```python
from build123d import *

# Parameters (mm, degrees)
F0_W      = 50.8
F0_H      = 50.8
F1_DEPTH  = 63.5
F3_DEPTH  = 12.7
F5_DEPTH  = 6.35
F6_DEPTH  = 50.8
F8_DEPTH  = 50.8
F10_DEPTH = 12.7


with BuildPart() as f1:
    # F0 (on Top) → F1 (new body)
    with BuildSketch(Plane.XY):
        Rectangle(F0_W, F0_H)
    extrude(amount=F1_DEPTH)

    # F2 (on face) → F3 (join)
    with BuildSketch(Plane.YZ.offset(25.4)):
        Polygon((-14.0506572952, 63.5), (0, 76.2), (0, 86.4714240594), (-36.0647195239, 53.8735228844), (-30.9551258806, 48.2205190104), (-25.4, 53.2416434461), (-25.4, 63.5), align=None)
        Polygon((-25.4, 53.2416434461), (-14.0506572952, 63.5), (-25.4, 63.5), align=None)
        Polygon((0, 86.4714240594), (0, 76.2), (14.0506572952, 63.5), (25.4, 63.5), (25.4, 53.2416434461), (31.0640838699, 48.1220349014), (36.1736775133, 53.7750387754), align=None)
        Polygon((25.4, 63.5), (14.0506572952, 63.5), (25.4, 53.2416434461), align=None)
    extrude(amount=F3_DEPTH)

    # F4 (on face) → F5 (join)
    with BuildSketch(Plane.YZ.offset(25.4)):
        Polygon((-14.0506572952, 63.5), (-25.4, 53.2416434461), (0, 25.1403288557), (25.4, 53.2416434461), (14.0506572952, 63.5), align=None)
        Polygon((0, 76.2), (-14.0506572952, 63.5), (14.0506572952, 63.5), align=None)
    extrude(amount=F5_DEPTH)

    # F6 (add): faces of the model
    f6_faces = [f1.faces().sort_by_distance(p)[0] for p in [
        (25.4, 0.0499832571, 67.5742219927),
        (25.4, 0.0499832571, 67.5742219927),
        (25.4, 0.0499832571, 67.5742219927),
    ]]
    extrude(f6_faces, amount=F6_DEPTH)

    # F7 (on face) → F8 (cut)
    with BuildSketch(Plane.YZ.offset(31.75)):
        with BuildLine():
            Line((-6.35, 53.2416434461), (6.35, 53.2416434461))
            ThreePointArc((6.35, 53.2416434461), (0, 59.5916434461), (-6.35, 53.2416434461))
        make_face()
        with BuildLine():
            ThreePointArc((-6.35, 53.2416434461), (0, 46.8916434461), (6.35, 53.2416434461))
            Line((6.35, 53.2416434461), (-6.35, 53.2416434461))
        make_face()
    extrude(amount=-F8_DEPTH, mode=Mode.SUBTRACT)

    # F9 (on face) → F10 (join)
    with BuildSketch(Plane.YZ.offset(31.75)):
        with BuildLine():
            ThreePointArc((1.27, 41.6503288557), (-0.8980256121, 42.5483544678), (0, 40.3803288557))
            ThreePointArc((0, 40.3803288557), (0.8980256121, 40.7523032436), (1.27, 41.6503288557))
        make_face()
    extrude(amount=F10_DEPTH)


solid = f1.part
```
Build history of the part. All positions in model axes, mm. A direction names the side the tool comes from. Coordinates: 2 decimals unless noted, no trailing zeros. Write each loop counter-clockwise with the first axis right and the second up, starting at its lowest first coordinate (ties: lowest second). Pieces come first, ordered by that corner, then holes.
1. Band-saw the part on D-D, the plane y = 9.5. Give the cut face in (x, z), and give its area (3 significant figures).
Answer block:
outline: (-25.4, 0) - (25.4, 0) - (25.4, 35.65) - (31.75, 35.65) - (31.75, 67.61) - (38.1, 67.61) - (38.1, 77.88) - (-25.4, 77.88) - close
area: 4,290 mm2
2. Drop flat-ended pins along their axis: pin 1 (1 mm diameter, centred on y = 5, z = 67, fed in from +X); pin 2 (10 mm diameter, centred on x = 4, z = 35, fed in from +Y); pin 3 (15 mm diameter, centred on y = -7, z = 63, fed in from +X). Give the stop position or say it passes through.
Answer block:
pin 1: stops at x = 31.75
pin 2: stops at y = 25.4
pin 3: stops at x = 38.1
3. Band-saw the part on A-A, the plane x = -15. Give the cut face in (y, z).
Answer block:
outline: (-36.06, 53.87) - (-30.96, 48.22) - (-25.4, 53.24) - (-25.4, 0) - (25.4, 0) - (25.4, 53.24) - (31.06, 48.12) - (36.17, 53.78) - (0, 86.47) - close; hole circle Ø12.7 at (0, 53.24)
4. Band-saw the part on B-B, the plane z = 31. Give the cut face in (x, y).
Answer block:
outline: (-25.4, -25.4) - (25.4, -25.4) - (25.4, -5.3) - (31.75, -5.3) - (31.75, 5.3) - (25.4, 5.3) - (25.4, 25.4) - (-25.4, 25.4) - close
5. Band-saw the part on C-C, the plane x = 28.5. Give the cut face in (y, z), and give its area (3 significant figures).
Answer block:
outline: (-36.06, 53.87) - (-30.96, 48.22) - (-25.4, 53.24) - (0, 25.14) - (25.4, 53.24) - (31.06, 48.12) - (36.17, 53.78) - (0, 86.47) - close; hole circle Ø12.7 at (0, 53.24)
area: 1,860 mm2
6. Pull direction Z, two halves, no side cores. Call faces 4 (the flat face through (-19.05, 0, 53)), 5 (the flat face through (0, 0, 0)), 6 (the flat face through (0, 25.4, 26)): released by +Z, released by -Z, zero draft, split by the parting line, or undercut.
Answer block:
face 4: undercut
face 5: released by -Z
face 6: zero draft
7. Drill centre lines: probe 1 along Y at (x, z) = (11.5, 52.5); probe 2 along X at (y, z) = (-16, 24). Where is each one in solid material? Low to high.
Answer block:
probe 1: y = -34.82 to -26.22, -25.4 to -6.31, 6.31 to 25.4, 26.22 to 35.02
probe 2: x = -25.4 to 25.4
8. 3-axis set-ups, long thin cutter, end or side, ignore diameter. For faces 1 (the flat face through (6.794, 33.583, 50.909)), 2 (the flat face through (28.53, 12.52, 38.99)), 3 (the cylindrical face through (6.706, 0.827, 46.946)): which of +Z, -Z, +X, -X, +Y, -Y reach the whole face in a straight line?
Answer block:
face 1: -Z, +X, -X, +Y
face 2: -Z, +X
face 3: +X
